The listing builds one solid part. Answer for the finished solid, in the listing's coordinates (mm). Face numbers are marked on the shaded views. A direction names the side the tool comes from. Round coordinates to 2 decimals unless told otherwise and drop trailing zeros. Loops run counter-clockwise (first coordinate to the right, second up) from the corner with the lowest first, then second, coordinate; pieces in that order, holes last. Notation, with made-up numbers: M -7.75,-33 L 29.25,-33 A27 ccw 29.25,-11 Z; hole C -22,63 d10. An arc over 180 degrees is marked long. Put each result on its own line as item: value. Start each with the question number.
(1) Section A-A, the plane z = 0 is taken. Determine the outline of the cut face in (x, y) (3 decimals).
(2) Determine the mould class of the marked faces 3, 4, 5 and 6 for opening direction Z: released by +Z, released by -Z, zero draft, split by the parting line, or undercut.
(3) Flat-ended cylindrical pins translate along their axes: P1, Ø4, axis at x = 4.5, z = -2.5, coming from the +Y side; P2, Ø12, axis at y = 0, z = 4, coming from the +X side; P3, Ø3, axis at x = 6, z = 8, coming from the +Y side; P4, Ø1, axis at x = 0, z = 9.5, coming from the +Y side. Find the tip coordinate at first contact, or state that the pin passes through.
(4) Section B-B, the plane y = 1.5 is taken. Determine the outline of the cut face in (x, z) (3 decimals), then the cut area to 3 significant figures.
(5) Section D-D, the plane x = 1.5 is taken. Determine the outline of the cut face in (y, z) (3 decimals), then the cut area to 3 significant figures.
(6) Which of the six approach directions +Z, -Z, +X, -X, +Y, -Y give full straight-line access (tool end or side, diameter ignored) to the marked faces 1 and 2?
(7) Straight lines are drawn through the part: line 1 (Y direction, x = 0.25, z = 0) (3 decimals); line 2 (Z direction, x = 0.5, y = 0); line 3 (Z direction, x = -0.25, y = 0). For each, find the intervals that lie inside material, in ascending order.
(8) Section C-C, the plane x = -1.25 is taken. Determine the outline of the cut face in (y, z).
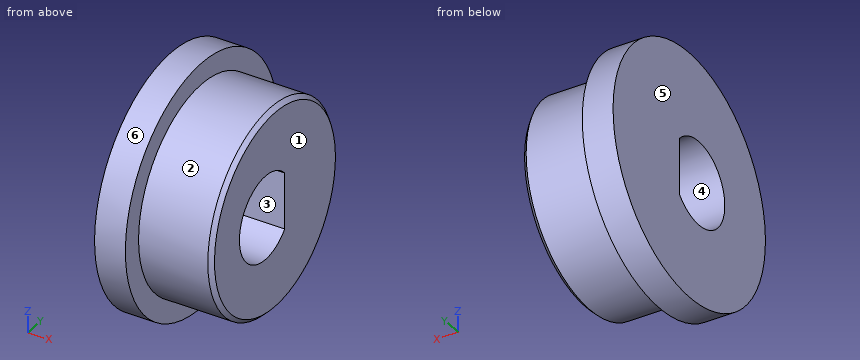
```python
from build123d import *

# Parameters (mm, degrees)
SKIZZE1_R                            = 9.925
AUFSATZ_LINEAR_AUSTRAGEN1_DEPTH      = 7.15
SKIZZE2_R                            = 12
AUFSATZ_LINEAR_AUSTRAGEN2_DEPTH      = 3
SCHNITT_LINEAR_AUSTRAGEN2_DEPTH      = 21.718892345
SCHNITT_LINEAR_AUSTRAGEN2_DEPTH_BACK = 21.718892345
FASE1_SIZE                           = 0.4


with BuildPart() as part:
    # Skizze1 → Aufsatz-Linear austragen1 (new body)
    with BuildSketch(Plane(origin=(0, 0, 0), x_dir=(0, 0, -1), z_dir=(1, 0, 0))):
        with Locations((0, 1.5)):
            Circle(SKIZZE1_R)
    extrude(amount=AUFSATZ_LINEAR_AUSTRAGEN1_DEPTH)

    # Skizze2 → Aufsatz-Linear austragen2 (add)
    with BuildSketch(Plane.ZY):
        with Locations((0, 1.5)):
            Circle(SKIZZE2_R)
    extrude(amount=AUFSATZ_LINEAR_AUSTRAGEN2_DEPTH)

    # Skizze3 → Schnitt-Linear austragen2 (cut, two sides: drawn at the far end of the back side and taken through both)
    with BuildSketch(Plane(origin=(7.15, 0, 0), x_dir=(0, 0, -1), z_dir=(1, 0, 0)).offset(-SCHNITT_LINEAR_AUSTRAGEN2_DEPTH_BACK)):
        with BuildLine():
            Line((-2.75, 3.04097024), (2.75, 3.04097024))
            ThreePointArc((2.75, 3.04097024), (0, -4.1), (-2.75, 3.04097024))
        make_face()
    extrude(amount=SCHNITT_LINEAR_AUSTRAGEN2_DEPTH + SCHNITT_LINEAR_AUSTRAGEN2_DEPTH_BACK, mode=Mode.SUBTRACT)

    # Fase1
    fase1_edges = [part.edges().sort_by_distance(p)[0] for p in [
        (7.15, 1.5, 9.925),
    ]]
    chamfer(fase1_edges, length=FASE1_SIZE)


solid = part.part
```
Recorded:
1. outline: M -3,-10.5 L 0,-10.5 L 0,-8.425 L 6.75,-8.425 L 7.15,-8.025 L 7.15,-4.1 L -3,-4.1 Z; M -3,3.041 L 7.15,3.041 L 7.15,11.025 L 6.75,11.425 L 0,11.425 L 0,13.5 L -3,13.5 Z
2. face 3: undercut
2. face 4: undercut
2. face 5: zero draft
2. face 6: split by the parting line
3. P1: stops at y = 11.41
3. P2: stops at x = 7.15
3. P3: stops at y = 9
3. P4: stops at y = 9.44
4. outline: M -3,-12 L 0,-12 L 0,-9.925 L 6.75,-9.925 L 7.15,-9.525 L 7.15,-3.816 L -3,-3.816 Z; M -3,3.816 L 7.15,3.816 L 7.15,9.525 L 6.75,9.925 L 0,9.925 L 0,12 L -3,12 Z
4. area: 136 mm²
5. outline: C 1.5,0 d19.85; hole M 3.041,-2.75 L 3.041,2.75 A4.1 ccw long Z
5. area: 261 mm²
6. face 1: +Z, -Z, +X, +Y, -Y
6. face 2: +X
7. line 1: y = -8.425 to -4.1, 3.041 to 11.425
7. line 2: z = -9.81 to -4.1, 4.1 to 9.81
7. line 3: z = -11.91 to -4.1, 4.1 to 11.91
8. outline: C 1.5,0 d24; hole M 3.04,-2.75 L 3.04,2.75 A4.1 ccw long Z
